from build123d import *

# Parameters (mm, degrees)
SKETCH1_W           = 8
SKETCH1_H           = 12
BOSS_EXTRUDE1_DEPTH = 150
LPATTERN1_COUNT     = 6
LPATTERN1_PITCH     = 25


with BuildPart() as part:
    # Sketch1 → Boss-Extrude1 (new body)
    with BuildSketch(Plane(origin=(0, 0, 0), x_dir=(0, 0, -1), z_dir=(1, 0, 0))):
        Rectangle(SKETCH1_W, SKETCH1_H)
    extrude(amount=BOSS_EXTRUDE1_DEPTH)

    # Sketch4 → Cut-Revolve1 (revolve, cut)
    with BuildSketch(Plane.ZY.offset(-11.75), mode=Mode.PRIVATE) as cut_revolve1_sk:
        Polygon((4, 0), (-4, 0), (-4, -1.75), (0, -1.75), (4, -3), align=None)
    cut_revolve1 = revolve(cut_revolve1_sk.sketch.rotate(Axis((11.75, 0, 4), (0, 0, -1)), 270), axis=Axis((11.75, 0, 4), (0, 0, -1)), mode=Mode.SUBTRACT)

    # LPattern1: Cut-Revolve1 ×6
    with Locations(*[(i * LPATTERN1_PITCH, 0, 0) for i in range(1, LPATTERN1_COUNT)]):
        add(cut_revolve1, mode=Mode.SUBTRACT)


solid = part.part
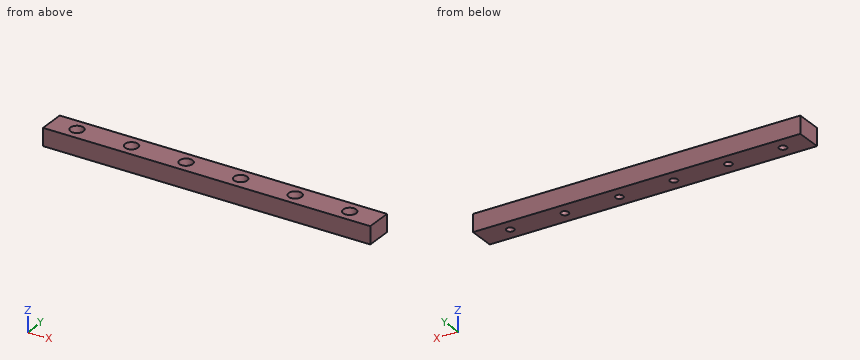
Design review of the part built by this model. Coordinates are the model's own, in mm. Give positions to 0.01 mm unless a question says otherwise; leave off trailing zeros. Loops run counter-clockwise (first coordinate to the right, second up) from the corner with the lowest first, then second, coordinate; pieces in that order, holes last. Notation, with made-up numbers: (-1, -17.75) - (6, -17.75) arc R19 ccw to (6, 5.25) - close; hole circle Ø10 at (18, 75.5). An arc over 180 degrees is marked (long way). Use CSV: the item, a comma, the result in double quotes. Start each with the question number.
1. Add section B-B (z = 1.25). State the section outline as (x, y) points.
2. Insertion check: P1, Ø3, axis at x = 11.75, y = 0, coming from the -Z side. The pin has a flat end and moves straight along its axis. Give the tip position at first contact, or say it passes through.
3. Add section A-A (x = 61.75). State the section outline as (y, z) points, plus the area to 3 significant figures.
4. Wall thickness on L1, parallel to Y at x = 136.75, z = -2.1; L2, parallel to Y at x = 112.5, z = -3.5: over which ranges is each line inside the solid? List them lowest first.
Results found:
1,outline,"(0, -6) - (150, -6) - (150, 6) - (0, 6) - close; hole circle Ø4.28 at (11.75, 0); hole circle Ø4.28 at (36.75, 0); hole circle Ø4.28 at (61.75, 0); hole circle Ø4.28 at (86.75, 0); hole circle Ø4.28 at (111.75, 0); hole circle Ø4.28 at (136.75, 0)"
2,P1,"passes through"
3,outline,"(-6, -4) - (-1.75, -4) - (-1.75, 0) - (-3, 4) - (-6, 4) - close; (1.75, -4) - (6, -4) - (6, 4) - (3, 4) - (1.75, 0) - close"
3,area,"63.0 mm²"
4,L1,"y = -6 to -1.75, 1.75 to 6"
4,L2,"y = -6 to -1.58, 1.58 to 6"
